Read the model definition and answer for the solid it produces. Units are mm, in the model's axes. Coordinates: 2 decimals unless noted, no trailing zeros. Write each loop counter-clockwise with the first axis right and the second up, starting at its lowest first coordinate (ties: lowest second). Pieces come first, ordered by that corner, then holes.
(1) The part is cut by section B-B, the plane z = 0. Determine the outline of the cut face in (x, y) (3 decimals), and give its area (3 significant figures).
(2) Given pin 1 (3 mm diameter, centred on x = 4, y = 4.5, fed in from +Z); pin 2 (2 mm diameter, centred on x = -6.05, z = -3.49, fed in from -Y); pin 3 (2 mm diameter, centred on y = 5.5, z = 6, fed in from -X), each flat-ended and moving along its own axis, determine where each tip first touches the part or whether it passes through.
(3) Straight lines are drawn through the part: line 1 along X through (y, z) = (6.25, -6.25); line 2 along Z through (x, y) = (6, 4.75); line 3 along X through (y, z) = (4, 2.5). For each, find the intervals that lie inside material, in ascending order.
(4) The part is cut by section C-C, the plane y = 3. State how many separate pieces and enclosed holes the cut face has, and give its area (3 significant figures).
(5) The part is cut by section D-D, the plane x = -7.5. Determine the outline of the cut face in (y, z), and give its area (3 significant figures).
(6) The part is cut by section A-A, the plane x = 0. Determine the outline of the cut face in (y, z) (3 decimals).
(7) Determine the mould class of faces 1 (the flat face through (0, 6.35, 0)), 2 (the cylindrical face through (5.822, 3.131, -0.366)), 3 (the cylindrical face through (7.559, 3.131, 5.796)) for opening direction X: pulls with the +X half, pulls with the -X half, needs draft (parallel to the pull), parting line crosses it, or undercut.
Autodesk Inventor part; units mm, degrees
ref_plane "YZ Plane" through (0, 0, 0) normal (1, 0, 0) x (0, 1, 0)
ref_plane "XZ Plane" through (0, 0, 0) normal (0, 1, 0) x (-1, 0, 0)
ref_plane "XY Plane" through (0, 0, 0) normal (0, 0, 1) x (1, 0, 0)
sketch "Sketch1" plane through (0, 0, 0) normal (0, 1, 0) x (-1, 0, 0)
  circle A0 centre (0, 0) radius 9.525
  dimension "d0" = 19.05
extrude "Extrusion1" add sketch "Sketch1" along normal blind 6.35
sketch "Sketch2" plane through (0, 6.35, 0) normal (0, 1, 0) x (1, 0, 0)
  point P0 (0, 0)
  point P1 (0, 6.985)
  dimension "d3" = 6.985
hole "Hole1" at (0, 6.35, -6.985) direction (0, -1, 0) diameter 2.4384 end through all
pattern_circular "Circular Pattern1" count 12 over 360 about axis through (0, 0, 0) along (0, 1, 0) of "Hole1"
properties part number "ferris_wheel_hub"
Computed:
1. outline: (-9.525, 0) - (-8.204, 0) - (-8.204, 6.35) - (-9.525, 6.35) - close; (-5.766, 0) - (5.766, 0) - (5.766, 6.35) - (-5.766, 6.35) - close; (8.204, 0) - (9.525, 0) - (9.525, 6.35) - (8.204, 6.35) - close
1. area: 90.0 mm2
2. pin 1: stops at z = 9.19
2. pin 2: passes through
2. pin 3: stops at x = -8.11
3. line 1: x = -7.19 to -4.7, -2.29 to -0.97, 0.97 to 2.29, 4.7 to 7.19
3. line 2: z = -7.4 to -4.71, -2.27 to -0.72, 0.72 to 2.27, 4.71 to 7.4
3. line 3: x = -9.19 to -6.76, -5.34 to 5.34, 6.76 to 9.19
4. separate pieces: 1
4. enclosed holes: 12
4. area: 229 mm2
5. outline: (0, -5.87) - (6.35, -5.87) - (6.35, -1.11) - (0, -1.11) - close; (0, 1.11) - (6.35, 1.11) - (6.35, 5.87) - (0, 5.87) - close
5. area: 60.5 mm2
6. outline: (0, -9.525) - (6.35, -9.525) - (6.35, -8.204) - (0, -8.204) - close; (0, -5.766) - (6.35, -5.766) - (6.35, 5.766) - (0, 5.766) - close; (0, 8.204) - (6.35, 8.204) - (6.35, 9.525) - (0, 9.525) - close
7. face 1: needs draft
7. face 2: undercut
7. face 3: parting line crosses it
